from build123d import *

# Parameters (mm, degrees)
SKETCH1_W             = 40
SKETCH1_H             = 22.7
BOSS_EXTRUDE1_DEPTH   = 6
F_4_CLEARANCE_HOLE1_D = 3.2639
F_3_0MM_DOWEL_HOLE1_D = 3


with BuildPart() as part:
    # Sketch1 → Boss-Extrude1 (new body)
    with BuildSketch(Plane.XY):
        Rectangle(SKETCH1_W, SKETCH1_H)
    extrude(amount=-BOSS_EXTRUDE1_DEPTH)

    # #4 Clearance Hole1 (through all)
    with Locations(Plane.XY):
        with Locations((-13.09, 0), (13.09, 0)):
            Hole(F_4_CLEARANCE_HOLE1_D / 2)

    # Ø3.0mm Dowel Hole1 (through all)
    with Locations(Plane.XY):
        with Locations((0, 0)):
            Hole(F_3_0MM_DOWEL_HOLE1_D / 2)


solid = part.part
Build history of the part. All positions in model axes, mm. Give positions to 0.01 mm unless a question says otherwise; leave off trailing zeros. Loops run counter-clockwise (first coordinate to the right, second up) from the corner with the lowest first, then second, coordinate; pieces in that order, holes last. Notation, with made-up numbers: (39, 4.25) -> (65, 4.25) arc R16 ccw to (65, 34.25) -> close; hole circle Ø4 at (-37, -5.5). An arc over 180 degrees is marked (long way). Answer in a Markdown table with one row per item.
Item 1: Slice it at A-A on y = 0. Write the cut outline in (x, z).
Findings below:
| item | result |
|---|---|
| outline | (-20, -6) -> (-14.72, -6) -> (-14.72, 0) -> (-20, 0) -> close; (-11.46, -6) -> (-1.5, -6) -> (-1.5, 0) -> (-11.46, 0) -> close; (1.5, -6) -> (11.46, -6) -> (11.46, 0) -> (1.5, 0) -> close; (14.72, -6) -> (20, -6) -> (20, 0) -> (14.72, 0) -> close |
Item 2: Slice it at B-B on x = 0. Write the cut outline in (y, z).
Findings below:
| item | result |
|---|---|
| outline | (-11.35, -6) -> (-1.5, -6) -> (-1.5, 0) -> (-11.35, 0) -> close; (1.5, -6) -> (11.35, -6) -> (11.35, 0) -> (1.5, 0) -> close |
Item 3: Flat gauge pin, fed straight in: P1, Ø2.5, axis at x = 0, y = 0, coming from the +Z side. Where does the tip first touch, or does it go through?
Findings below:
| item | result |
|---|---|
| P1 | passes through |
Item 4: Probe line 1 along Y through (x, z) = (13.09, -2.5); line 2 along Y through (x, z) = (0, -4.4). List the from-to ranges inside material, lowest first. Write a range as [from, to].
Findings below:
| item | result |
|---|---|
| line 1 | y = [-11.35, -1.63], [1.63, 11.35] |
| line 2 | y = [-11.35, -1.5], [1.5, 11.35] |
Item 5: Slice it at C-C on z = -4.4. Write the cut outline in (x, y).
Findings below:
| item | result |
|---|---|
| outline | (-20, -11.35) -> (20, -11.35) -> (20, 11.35) -> (-20, 11.35) -> close; hole circle Ø3.26 at (-13.09, 0); hole circle Ø3 at (0, 0); hole circle Ø3.26 at (13.09, 0) |
Item 6: Mould opens along Y. For faces 1 (the cylindrical face through (1.5, 0.07, -3.04)), 2 (the flat face through (0, -11.35, -3)), 3 (the cylindrical face through (-12.736, -1.593, -3.042)), 4 (the flat face through (-20, 0, -3)) say: pulls with the +Y half, pulls with the -Y half, needs draft (parallel to the pull), parting line crosses it, or undercut.
Findings below:
| item | result |
|---|---|
| face 1 | undercut |
| face 2 | pulls with the -Y half |
| face 3 | undercut |
| face 4 | needs draft |
